Verification items for this drawing (mm, ordinates from the low corner). A direction names the side the tool comes from. Round coordinates to 2 decimals unless told otherwise and drop trailing zeros. Loops run counter-clockwise (first coordinate to the right, second up) from the corner with the lowest first, then second, coordinate; pieces in that order, holes last. Notation, with made-up numbers: (46, 24.25) -> (59, 24.25) arc R20 cw to (59, 52.25) -> close; hole circle Ø8 at (46.5, -6). An arc over 180 degrees is marked (long way). Use a Markdown table: item, result. Add a question column.
Q1. Set-up check for the marked faces 1 and 2: record each of +Z, -Z, +X, -X, +Y, -Y from which the full face is reachable in a straight line by a thin tool's end or side.
Q2. Release check for a two-part mould opening along X. For the marked faces 3, 4 and 5 record: released by +X, released by -X, zero draft, split by the parting line, or undercut.
Q3. Sectioned sample at D-D, the plane z = 6. Enter the section's corners in (x, y), then the cut area to 3 significant figures.
Q4. Sectioned sample at C-C, the plane z = 8.75. Enter the section's corners in (x, y), then the cut area to 3 significant figures.
Q5. Gauge pin test, flat ends, axial feed: P1, Ø2, axis at x = 12.5, y = 0.5, coming from the -Z side; P2, Ø1.5, axis at x = 22.5, y = 24.5, coming from the -Z side. Record the tip position at first contact, or that the pin passes through.
Q6. Material ranges on L1, parallel to X at y = 3.5, z = 11; L2, parallel to Y at x = 14.8, z = 12.5; L3, parallel to Y at x = 14.5, z = 10.25, recorded low to high.
Q7. Sectioned sample at A-A, the plane y = 26.5. Enter the section's corners in (x, z), then the cut area to 3 significant figures.
Q8. Sectioned sample at B-B, the plane x = 14.8. Enter the section's corners in (y, z).
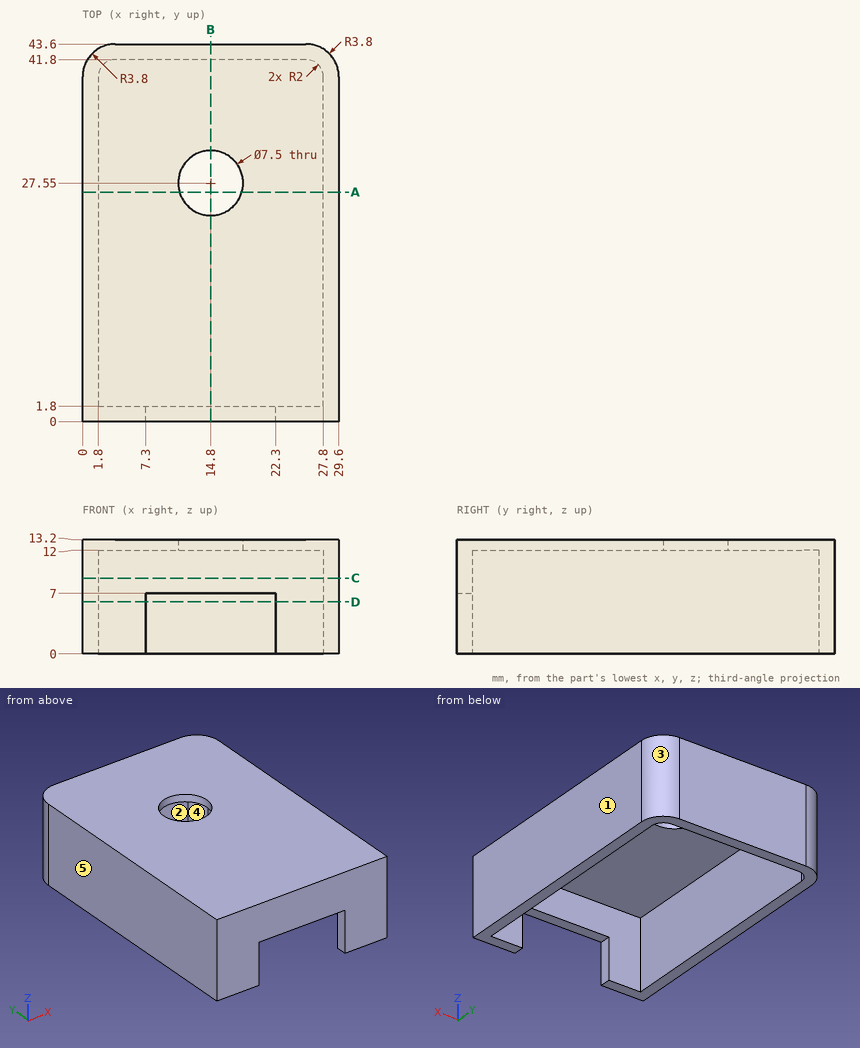
Values:
| question | item | result |
|---|---|---|
| 1 | face 1 | +Z, -Z, +X, +Y, -Y |
| 1 | face 2 | -Z |
| 2 | face 3 | released by +X |
| 2 | face 4 | undercut |
| 2 | face 5 | released by -X |
| 3 | outline | (0, 0) -> (7.3, 0) -> (7.3, 1.8) -> (1.8, 1.8) -> (1.8, 39.8) arc R2 cw to (3.8, 41.8) -> (25.8, 41.8) arc R2 cw to (27.8, 39.8) -> (27.8, 1.8) -> (22.3, 1.8) -> (22.3, 0) -> (29.6, 0) -> (29.6, 39.8) arc R3.8 ccw to (25.8, 43.6) -> (3.8, 43.6) arc R3.8 ccw to (0, 39.8) -> close |
| 3 | area | 219 mm^2 |
| 4 | outline | (0, 0) -> (29.6, 0) -> (29.6, 39.8) arc R3.8 ccw to (25.8, 43.6) -> (3.8, 43.6) arc R3.8 ccw to (0, 39.8) -> close; hole (1.8, 1.8) -> (27.8, 1.8) -> (27.8, 39.8) arc R2 ccw to (25.8, 41.8) -> (3.8, 41.8) arc R2 ccw to (1.8, 39.8) -> close |
| 4 | area | 246 mm^2 |
| 5 | P1 | z = 7 |
| 5 | P2 | z = 12 |
| 6 | L1 | 0 to 1.8, 27.8 to 29.6 |
| 6 | L2 | 0 to 23.8, 31.3 to 43.6 |
| 6 | L3 | 0 to 1.8, 41.8 to 43.6 |
| 7 | outline | (0, 0) -> (1.8, 0) -> (1.8, 12) -> (11.2, 12) -> (11.2, 13.2) -> (0, 13.2) -> close; (18.4, 12) -> (27.8, 12) -> (27.8, 0) -> (29.6, 0) -> (29.6, 13.2) -> (18.4, 13.2) -> close |
| 7 | area | 70.1 mm^2 |
| 8 | outline | (0, 7) -> (1.8, 7) -> (1.8, 12) -> (23.8, 12) -> (23.8, 13.2) -> (0, 13.2) -> close; (31.3, 12) -> (41.8, 12) -> (41.8, 0) -> (43.6, 0) -> (43.6, 13.2) -> (31.3, 13.2) -> close |
